Can you work these out from the model? Positions are in its coordinate system, mm. Give positions to 0.01 mm unless a question says otherwise; leave off trailing zeros. Order: outer loops, then holes, each group sorted by start corner. A loop starts at its lowest first (then second) coordinate and runs counter-clockwise, first axis right, second up. Notation, with made-up numbers: M 6.25,-26.5 L 24.25,-26.5 A13 ccw 24.25,-1.5 Z; hole C 79.5,36.25 d5. An arc over 180 degrees is marked long. Write each question's results on one line, items separated by ' | '.
from build123d import *

# Parameters (mm, degrees)
F0_W       = 14
F0_H       = 40
F0_R       = 3
F1_DEPTH   = 2
F2_SIZE2   = 1
F2_SIZE    = 3
F2_2_SIZE2 = 1
F2_2_SIZE  = 3
F3_R       = 3


with BuildPart() as f1:
    # F0 (on Front) → F1 (new body, symmetric)
    with BuildSketch(Plane.XZ):
        Rectangle(F0_W, F0_H)
        Circle(F0_R, mode=Mode.SUBTRACT)
    extrude(amount=F1_DEPTH, both=True)

    # F2
    f2_edges = [f1.edges().sort_by_distance(p)[0] for p in [
        (0, -2, 20),
        (0, -2, -20),
    ]]
    f2_side = f1.faces().sort_by_distance((6.576208, -2, 0))[0]
    chamfer(f2_edges, length=F2_SIZE, length2=F2_SIZE2, reference=f2_side)

    # F2#2
    f2_2_edges = [f1.edges().sort_by_distance(p)[0] for p in [
        (0, 2, 20),
        (0, 2, -20),
    ]]
    f2_2_side = f1.faces().sort_by_distance((6.576208, 2, 0))[0]
    chamfer(f2_2_edges, length=F2_2_SIZE, length2=F2_2_SIZE2, reference=f2_2_side)

    # F3
    f3_edges = [f1.edges().sort_by_distance(p)[0] for p in [
        (7, 0, 20),
        (-7, 0, 20),
        (7, 0, -20),
        (-7, 0, -20),
    ]]
    fillet(f3_edges, radius=F3_R)


solid = f1.part
(1) Imagine slicing it at A-A, the plane x = 0. Write out the boundary of the cut face in (y, z), plus the area to 3 significant figures.
Data:
outline: M -2,-17 L -1,-20 L 1,-20 L 2,-17 L 2,-3 L -2,-3 Z; M -2,3 L 2,3 L 2,17 L 1,20 L -1,20 L -2,17 Z | area: 130 mm2
(2) We'd pull the mould along X, two halves only. Please class faces 1 (the face through (-3, 0, 0)), 2 (the face through (-0.1, 1.5, 18.5)), 3 (the face through (-7, 0, 0)): +X half, -X half, draft (parallel to the pull), parting line (faces both ways), or undercut.
Data:
face 1: undercut | face 2: draft | face 3: -X half
(3) Imagine slicing it at C-C, the plane y = 0.35. Write out the boundary of the cut face in (x, z).
Data:
outline: M -7,-17 A3 ccw -4,-20 L 4,-20 A3 ccw 7,-17 L 7,17 A3 ccw 4,20 L -4,20 A3 ccw -7,17 Z; hole C 0,0 d6
(4) Imagine slicing it at B-B, the plane z = 0. Write out the boundary of the cut face in (x, y).
Data:
outline: M -7,-2 L -3,-2 L -3,2 L -7,2 Z; M 3,-2 L 7,-2 L 7,2 L 3,2 Z
(5) Imagine slicing it at D-D, the plane x = 5. Write out the boundary of the cut face in (y, z), plus the area to 3 significant figures.
Data:
outline: M -2,-17 L -1.06,-19.83 L 1.06,-19.83 L 2,-17 L 2,17 L 1.06,19.83 L -1.06,19.83 L -2,17 Z | area: 153 mm2
(6) Will this pin go through, and if not, where does the flat tip stop? P1, Ø5, axis at x = 0, z = 0, coming from the +Y side.
Data:
P1: passes through
(7) I need wall thicknesses on L1, parallel to Z at x = 0, y = -0.65; L2, parallel to X at y = 1.65, z = -0.5; L3, parallel to Z at x = -2, y = 0.75. Which ranges of each line are inside material? Lowest first, please. Write a range as from..to.
Data:
L1: z = -20..-3, 3..20 | L2: x = -7..-2.96, 2.96..7 | L3: z = -20..-2.24, 2.24..20
